Here's how the part is built. I have some questions about the finished solid (model axes, mm). A direction names the side the tool comes from. Coordinates: 2 decimals unless noted, no trailing zeros. Write each loop counter-clockwise with the first axis right and the second up, starting at its lowest first coordinate (ties: lowest second). Pieces come first, ordered by that corner, then holes. Notation, with made-up numbers: (18.25, 84.5) -> (65.25, 84.5) arc R14 cw to (65.25, 102.5) -> close; hole circle Ø2 at (-20, -40). An arc over 180 degrees is marked (long way). Answer in a Markdown table with one row per item. Add a question column.
from build123d import *
from OCP.BRepFilletAPI import BRepFilletAPI_MakeChamfer

# Parameters (mm, degrees)
SKETCH1_W       = 20
SKETCH1_H       = 2.5
SKETCH1_W_2     = 13.5
SKETCH1_H_2     = 1.5
SKETCH1_W_3     = 1
SKETCH1_H_3     = 4
CHAMFER1_SIZE   = 1.5
CHAMFER1_SIZE2  = 3.216760381
CHAMFER2_SIZE   = 1.732050808
CHAMFER2_SIZE_2 = 1
FILLET6_R       = 2
CHAMFER3_SIZE   = 1
CHAMFER4_SIZE   = 0.7
SKETCH3_W       = 2
SKETCH3_H       = 1.4
SKETCH3_3_W     = 2
SKETCH3_3_H     = 1.4
SKETCH3_3_W_2   = 0.7
SKETCH3_3_H_2   = 2
REVOLVE3_ANGLE  = 355
CHAMFER5_SIZE   = 0.5


# Some blends are built 0.0001 mm under size
with BuildPart() as part:
    # Sketch1 → Revolve1 (revolve)
    with BuildSketch(Plane.XY, mode=Mode.PRIVATE) as revolve1_sk:
        with BuildLine():
            ThreePointArc((-20, 2.5), (-20.35, 2.85), (-20, 3.2))
            Line((-20, 3.2), (-20, 6.2))
            Line((-20, 6.2), (-24, 6.2))
            Line((-24, 6.2), (-24, 0))
            Line((-24, 0), (-20, 0))
            Line((-20, 0), (-20, 2.5))
        make_face()
        with BuildLine():
            Line((-20, 6.2), (-20, 3.2))
            add(Edge.make_bspline(
                [(-20, 3.2), (-17.980801876, 2.682507767), (-14.91231446, 2.835315185), (-10.877832782, 3.989364254), (-6.922969843, 2.860615153), (-3.936379553, 2.67369733), (-2, 3.2)],
                knots=[0, 0, 0, 0, 0.33680166, 0.506831372, 0.676362633, 1, 1, 1, 1], degree=3))
            Line((-2, 3.2), (-2, 6.2))
            Line((-2, 6.2), (-4, 6.2))
            Line((-4, 6.2), (-20, 6.2))
        make_face()
        with Locations((-10, 1.25)):
            Rectangle(SKETCH1_W, SKETCH1_H)
        Polygon((-4, 6.6), (-4, 6.2), (-2, 6.2), (-2, 14.2), (-2, 18.2), (-4, 18.2), (-4, 8.1), align=None)
        with Locations((-10.75, 7.35)):
            Rectangle(SKETCH1_W_2, SKETCH1_H_2)
        with Locations((-1.5, 16.2)):
            Rectangle(SKETCH1_W_3, SKETCH1_H_3)
    revolve(revolve1_sk.sketch.rotate(Axis((0, 0, 0), (0, 1, 0)), 270), axis=Axis((0, 0, 0), (0, 1, 0)))

    # Chamfer1: one chamfer whose edges measure the first distance from different faces: ONE call of the kernel's chamfer builder (chamfer() names one face for all edges)
    chamfer1_edges_1 = [part.edges().sort_by_distance(p)[0] for p in [
        (0, 0, 24),
    ]]
    chamfer1_side_1 = [part.faces().sort_by_distance(p)[0] for p in [
        (0, 3.1, 24),
    ]]
    chamfer1_edges_2 = [part.edges().sort_by_distance(p)[0] for p in [
        (0, 6.2, 24),
    ]]
    chamfer1_side_2 = [part.faces().sort_by_distance(p)[0] for p in [
        (0, 6.2, 23.32117749),
    ]]
    chamfer1 = BRepFilletAPI_MakeChamfer(part.part.solid().wrapped)
    for e in chamfer1_edges_1:
        chamfer1.Add(CHAMFER1_SIZE, CHAMFER1_SIZE2, e.wrapped, chamfer1_side_1[0].wrapped)  # the first distance lies on this face
    for e in chamfer1_edges_2:
        chamfer1.Add(CHAMFER1_SIZE, CHAMFER1_SIZE2, e.wrapped, chamfer1_side_2[0].wrapped)  # the first distance lies on this face
    add(Compound.cast(chamfer1.Shape()), mode=Mode.REPLACE)

    # Chamfer2
    # the kernel refuses this chamfer: 1.732050808, 1 mm, written as the material it adds along each edge
    with BuildSketch(Plane(origin=(0, 6.2, 0), x_dir=(0, 0, -1), z_dir=(1, 0, 0))) as chamfer2_piece_1:
        Polygon((4 + CHAMFER2_SIZE, 0), (4, CHAMFER2_SIZE_2), (4, 0), align=None)
    revolve(axis=Axis((0, 6.2, 0), (0, 1, 0)))

    # Fillet6
    fillet6_edges = [part.edges().sort_by_distance(p)[0] for p in [
        (0, 1.5, 24),
    ]]
    fillet(fillet6_edges, radius=FILLET6_R)

    # Chamfer3
    chamfer3_edges = [part.edges().sort_by_distance(p)[0] for p in [
        (0, 18.2, 1),
        (0, 14.2, 2),
    ]]
    chamfer(chamfer3_edges, length=CHAMFER3_SIZE - 0.0001)  # a hair under: the kernel refuses the full size

    # Chamfer4
    chamfer4_edges = [part.edges().sort_by_distance(p)[0] for p in [
        (0, 8.1, 17.5),
    ]]
    chamfer(chamfer4_edges, length=CHAMFER4_SIZE)

    # Sketch3 → Revolve2 (revolve)
    with BuildSketch(Plane.XY, mode=Mode.PRIVATE) as revolve2_sk:
        Polygon((0, 1), (0, -1.9), (-2, -1.9), (-2, -0.4), (-2, 1), align=None)
        with Locations((-3, 0.3)):
            Rectangle(SKETCH3_W, SKETCH3_H)
        Polygon((-2, -1.9), (-2, -0.4), (-4, -0.4), (-22.8, -0.4), (-23.5, -0.4), (-24, -0.4), (-24, -1.9), align=None)
    revolve(revolve2_sk.sketch.rotate(Axis((0, 0, 0), (0, 1, 0)), 270), axis=Axis((0, 0, 0), (0, 1, 0)))

    # Sketch3<3> → Revolve3 (revolve)
    with BuildSketch(Plane.XY):
        with Locations((-3, 0.3)):
            Rectangle(SKETCH3_3_W, SKETCH3_3_H)
        Polygon((0, 1), (-2, 1), (-2, -0.4), (-2, -1.9), (0, -1.9), align=None)
        Polygon((-2, -1.9), (-2, -0.4), (-4, -0.4), (-22.8, -0.4), (-23.5, -0.4), (-24, -0.4), (-24, -1.9), align=None)
        with Locations((-23.15, 0.6)):
            Rectangle(SKETCH3_3_W_2, SKETCH3_3_H_2)
    revolve(axis=Axis((0, 1, 0), (0, -1, 0)), revolution_arc=REVOLVE3_ANGLE)

    # Chamfer5
    chamfer5_edges = [part.edges().sort_by_distance(p)[0] for p in [
        (0, -1.9, 24),
    ]]
    chamfer(chamfer5_edges, length=CHAMFER5_SIZE)


solid = part.part
Q1. If we mould it in two halves opening along Z, with no side actions, what happens to faces 1 (the flat face through (0, -1.9, 0)), 2 (the conical face through (-6.79, 6, -21.55)), 3 (the flat face through (0, 2.5, 0))? For each: pulls with the +Z half, pulls with the -Z half, needs draft (parallel to the pull), parting line crosses it, or undercut.
Q2. I'm going to push flat-ended pins straight in: P1, Ø6, axis at y = 1.5, z = 14.5, coming from the +X side; P2, Ø1.5, axis at x = 4.5, y = 2, coming from the +Z side; P3, Ø5, axis at x = -5, y = 13.5, coming from the -Z side. Where does each tip first touch, or does it pass through?
Q3. I need wall thicknesses on line 1 (Y direction, x = 1, z = -16); line 2 (Y direction, x = -2.5, z = -7); line 3 (Z direction, x = -2, y = 0.25). Which ranges of each line are inside material? Lowest first, please. Write a range as [from, to].
Q4. For faces 4 (the cylindrical face through (23.41, 0.54, -2.04)), 5 (the cylindrical face through (-7.21, -0.91, -22.89)), 6 (the cylindrical face through (1, 16, 0)), which set-ups out of +Z, -Z, +X, -X, +Y, -Y let a thin tool reach every point of the face, with its end or its side?
Q5. Imagine slicing it at B-B on z = -8.5. State how many separate pieces and enclosed holes the cut face has, plus the area to 3 significant figures.
Q6. Imagine slicing it at A-A on y = 15.75. Please give me the cut outline in (x, z), plus the area to 3 significant figures.
Result sheet:
| question | item | result |
|---|---|---|
| 1 | face 1 | needs draft |
| 1 | face 2 | parting line crosses it |
| 1 | face 3 | undercut |
| 2 | P1 | stops at x = 20.95 |
| 2 | P2 | stops at z = 23.66 |
| 2 | P3 | stops at z = -3.12 |
| 3 | line 1 | y = [-1.9, -0.4], [0, 2.5], [2.89, 6.2], [6.6, 8.1] |
| 3 | line 2 | y = [-1.9, -0.4], [0, 2.5], [3.12, 6.2], [6.6, 8.1] |
| 3 | line 3 | z = [-23.41, -22.71], [-21.23, 21.23], [22.71, 23.41] |
| 4 | face 4 | none |
| 4 | face 5 | +Y, -Y |
| 4 | face 6 | +Y |
| 5 | separate pieces | 2 |
| 5 | enclosed holes | 2 |
| 5 | area | 353 mm^2 |
| 6 | outline | circle Ø8 at (0, 0); hole circle Ø2 at (0, 0) |
| 6 | area | 47.1 mm^2 |
